Here's how the part is built. I have some questions about the finished solid (model axes, mm). Give positions to 0.01 mm unless a question says otherwise; leave off trailing zeros. Write each loop counter-clockwise with the first axis right and the second up, starting at its lowest first coordinate (ties: lowest second). Pieces come first, ordered by that corner, then holes. Notation, with made-up numbers: (42, 56) -> (98, 56) arc R16 ccw to (98, 85) -> close; hole circle Ø8 at (29.25, 46.5). An arc over 180 degrees is marked (long way). Use one line per item in the form item = value.
Autodesk Inventor part; units mm, degrees
ref_plane "YZ Plane" through (0, 0, 0) normal (1, 0, 0) x (0, 1, 0)
ref_plane "XZ Plane" through (0, 0, 0) normal (0, 1, 0) x (-1, 0, 0)
ref_plane "XY Plane" through (0, 0, 0) normal (0, 0, 1) x (1, 0, 0)
sketch "Sketch1" plane through (0, 0, 0) normal (0, 1, 0) x (-1, 0, 0)
  line L0 (-2.9393, 4) -> (2.9393, 4)
  line L1 (4, 2.9393) -> (4, -2.9393)
  line L2 (2.9393, -4) -> (-2.9393, -4)
  line L3 (-4, -2.9393) -> (-4, 2.9393)
  circle A0 centre (0, 0) radius 2.15
  line L4 (-2.9393, 4) -> (-6.75, 7.8107)
  line L5 (-7.8107, 6.75) -> (-4, 2.9393)
  line L6 (4, -2.9393) -> (7.8107, -6.75)
  line L7 (-10, 10) -> (-2.5, 10)
  line L8 (2.5, 10) -> (10, 10)
  line L9 (10, -10) -> (2.5, -10)
  line L10 (-2.5, -10) -> (-10, -10)
  line L11 (10, 10) -> (10, 2.5)
  line L12 (10, -2.5) -> (10, -10)
  line L13 (-10, -10) -> (-10, -2.5)
  line L14 (-10, 2.5) -> (-10, 10)
  line L15 (-8.5, 2.5) -> (-8.5, 6.75)
  line L16 (-6.75, 8.5) -> (-2.5, 8.5)
  line L17 (2.5, 10) -> (2.5, 8.5)
  line L18 (10, 2.5) -> (8.5, 2.5)
  line L19 (10, -2.5) -> (8.5, -2.5)
  line L20 (2.5, -8.5) -> (2.5, -10)
  line L21 (-2.5, -8.5) -> (-2.5, -10)
  line L22 (-8.5, -2.5) -> (-10, -2.5)
  line L23 (-8.5, 2.5) -> (-10, 2.5)
  line L24 (-2.5, 10) -> (-2.5, 8.5)
  line L25 (-7.8107, 6.75) -> (-8.5, 6.75)
  line L26 (-6.75, 8.5) -> (-6.75, 7.8107)
  line L27 (6.75, 8.5) -> (6.75, 7.8107)
  line L28 (8.5, 6.75) -> (7.8107, 6.75)
  line L29 (8.5, 6.75) -> (8.5, 2.5)
  line L30 (2.5, 8.5) -> (6.75, 8.5)
  line L31 (6.75, 7.8107) -> (2.9393, 4)
  line L32 (7.8107, 6.75) -> (4, 2.9393)
  line L33 (2.9393, -4) -> (6.75, -7.8107)
  line L34 (8.5, -2.5) -> (8.5, -6.75)
  line L35 (6.75, -8.5) -> (2.5, -8.5)
  line L36 (8.5, -6.75) -> (7.8107, -6.75)
  line L37 (6.75, -7.8107) -> (6.75, -8.5)
  line L38 (-2.5, -8.5) -> (-6.75, -8.5)
  line L39 (-2.9393, -4) -> (-6.75, -7.8107)
  line L40 (-8.5, -6.75) -> (-8.5, -2.5)
  line L41 (-4, -2.9393) -> (-7.8107, -6.75)
  line L42 (-6.75, -7.8107) -> (-6.75, -8.5)
  line L43 (-7.8107, -6.75) -> (-8.5, -6.75)
  dimension "d0" = 20
  dimension "d1" = 20
  dimension "d26" = 1.5
  dimension "d27" = 1.5
  dimension "d32" = 7.5
  dimension "d33" = 5
  dimension "d34" = 7.5
  dimension "d35" = 7.5
  dimension "d40" = 6
  dimension "d41" = 13.5
extrude "Extrusion1" add sketch "Sketch1" along normal blind 160
chamfer "Chamfer1" distance 0.5 angle 45 12 edges at (-10, 80, 2.5) (-10, 80, -2.5) (-2.5, 80, 10) (2.5, 80, 10) (10, 80, 2.5) (10, 80, -2.5) (2.5, 80, -10) (-2.5, 80, -10) (-10, 80, 10) (-10, 80, -10) (10, 80, -10) (10, 80, 10)
properties part number "2020 Extrusion 160mm" material "Aluminum 6061"
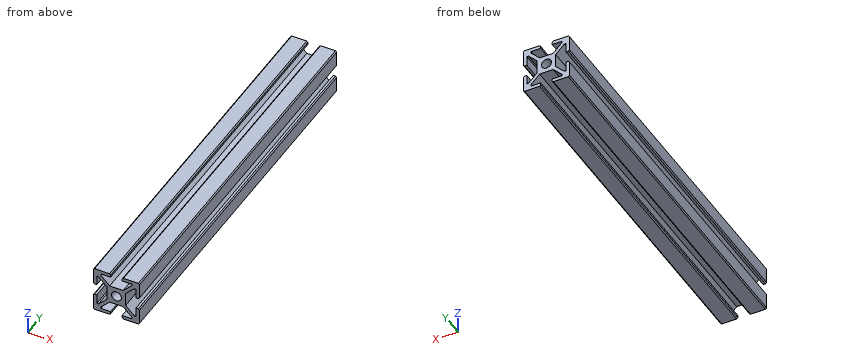
Q1. I want a section at A-A, the plane z = 0. Write out the boundary of the cut face in (x, y).
Result set:
outline = (-4, 0) -> (-2.15, 0) -> (-2.15, 160) -> (-4, 160) -> close; (2.15, 0) -> (4, 0) -> (4, 160) -> (2.15, 160) -> close
Q2. Will these pins go through, and if not, where does the flat tip stop? pin 1 Ø6 at (x, z) = (1.5, -2) entering from -Y; pin 2 Ø1.5 at (y, z) = (121.5, -2) entering from -X; pin 3 Ø1.8 at (y, z) = (65.5, 0) entering from +X; pin 4 Ø1.8 at (x, y) = (1, 116) entering from +Z.
Result set:
pin_1 = 0
pin_2 = -9.75
pin_3 = 4
pin_4 = 4
Q3. I want a section at B-B, the plane x = 0. Write out the boundary of the cut face in (y, z).
Result set:
outline = (0, -4) -> (160, -4) -> (160, -2.15) -> (0, -2.15) -> close; (0, 2.15) -> (160, 2.15) -> (160, 4) -> (0, 4) -> close
Q4. If I drill on line 1 along Z through (x, y) = (0, 47); line 2 along X through (y, z) = (80.5, -6); line 3 along X through (y, z) = (26.5, 5.75), over which ranges is the centre line in solid material (lowest first)? Write a range as from..to.
Result set:
line_1 = -4..-2.15, 2.15..4
line_2 = -10..-8.5, -7.06..-4.94, 4.94..7.06, 8.5..10
line_3 = -10..-8.5, -6.81..-4.69, 4.69..6.81, 8.5..10
